Autodesk Fusion 360 part; units mm, degrees
sketch "Sketch1" plane through (0, 0, 0) normal (0, 0, 1) x (1, 0, 0)
  circle A0 centre (0, 0) radius 25
  circle A1 centre (0, 0) radius 28
  dimension "d4" = 50
  dimension "d5" = 56
extrude "Extrude1" add sketch "Sketch1" along normal blind 3 contours A0
extrude "Extrude2" add sketch "Sketch1" along normal blind 60
chamfer "Chamfer2" distance 3 angle 45 1 edges at (-26.1052, -10.1252, 0)
move_face "OffsetFaces1" offset -0.5 1 faces at (24.8758, -2.4892, 22)
chamfer "Chamfer3" distance 3 angle 45 1 edges at (-23.7743, -9.2212, 3)
chamfer "Chamfer4" distance 2.5 angle 45 1 edges at (-23.7743, 9.2212, 60)
equation "wall_thinkness = 3 mm"
equation "pot_height = 60 mm"
equation "pot_diameter = 50 mm"
equation "d4 = pot_diameter"
equation "d5 = pot_diameter + ( 2 * wall_thinkness )"
equation "d6 = wall_thinkness"
equation "d8 = pot_height"
equation "pot_bottom_outer_fillet = 10 mm"
equation "pot_finger_cutout_width = 20 mm"
equation "pot_finger_cutout_height = 7 mm"
Can you work these out from the model? Positions are in its coordinate system, mm. A direction names the side the tool comes from. Give positions to 0.01 mm unless a question says otherwise; leave off trailing zeros. Loops run counter-clockwise (first coordinate to the right, second up) from the corner with the lowest first, then second, coordinate; pieces in that order, holes last. Notation, with made-up numbers: M 0,48.5 L 38,48.5 A19 cw 38,58.5 Z; hole C 43,43 d1. An arc over 180 degrees is marked long. One line per item, written item: value.
1) I'm going to push flat-ended pins straight in: pin 1 (2 mm diameter, centred on y = 7, z = 43, fed in from -X); pin 2 (4 mm diameter, centred on x = 7, z = 48.5, fed in from -Y); pin 3 (12 mm diameter, centred on x = -17.5, y = 8, fed in from +Z). Where does each tip first touch, or does it pass through?
Geometry check:
pin 1: stops at x = -27.35
pin 2: stops at y = -27.55
pin 3: stops at z = 5.74
2) Thinking about a two-plate mould opening in Y: for faces 1 (the face through (0, 0, 0)), 2 (the face through (-5.46, -24.59, 0.19)), 3 (the face through (0, 0, 3)), which applies, +Y half, -Y half, draft (parallel to the pull), parting line (faces both ways), or undercut?
Geometry check:
face 1: draft
face 2: parting line
face 3: undercut
3) Imagine slicing it at B-B on z = 39. Write out the boundary of the cut face in (x, y), and give its area (3 significant figures).
Geometry check:
outline: C 0,0 d56; hole C 0,0 d51
area: 420 mm²
4) On a 3-axis mill with a long thin cutter (end or side, diameter ignored), from which of +Z, -Z, +X, -X, +Y, -Y can I reach the whole of each face in a straight line? I mean faces 4 (the face through (-5.5, 24.9, 31.4)), 5 (the face through (25.865, 10.724, 31.101)). Say none if no direction works.
Geometry check:
face 4: +Z
face 5: +Z, -Z
5) Please list where these lines run through material, in increasing order: line 1 (Y direction, x = 0, z = 22); line 2 (X direction, y = -5.5, z = 53).
Geometry check:
line 1: y = -28 to -25.5, 25.5 to 28
line 2: x = -27.45 to -24.9, 24.9 to 27.45
